```python
from build123d import *

# Parameters (mm, degrees)
SKETCH5_W           = 101.6
SKETCH5_H           = 101.6
SKETCH5_W_2         = 20.32
SKETCH5_H_2         = 20.32
BOSS_EXTRUDE1_DEPTH = 228.6
SKETCH6_R           = 41.91
CUT_EXTRUDE1_DEPTH  = 127
SKETCH5_3_W         = 20.32
SKETCH5_3_H         = 20.32
CUT_EXTRUDE2_DEPTH  = 25.4
CUT_EXTRUDE3_DEPTH  = 76.2
SKETCH9_R           = 7.62
CUT_EXTRUDE4_DEPTH  = 56.642


with BuildPart() as part:
    # Sketch5 → Boss-Extrude1 (new body)
    # profile 1 of 5: a face of its own
    with BuildSketch(Plane(origin=(0, 0, 0), x_dir=(1, 0, 0), z_dir=(0, 1, 0))):
        with Locations((50.8, 50.8)):
            Rectangle(SKETCH5_W, SKETCH5_H)
        with Locations((16.51, 15.457317153)):
            Rectangle(SKETCH5_W_2, SKETCH5_H_2, mode=Mode.SUBTRACT)
        with Locations((85.09, 15.457317153)):
            Rectangle(SKETCH5_W_2, SKETCH5_H_2, mode=Mode.SUBTRACT)
        with Locations((85.09, 85.09)):
            Rectangle(SKETCH5_W_2, SKETCH5_H_2, mode=Mode.SUBTRACT)
        with Locations((16.51, 85.09)):
            Rectangle(SKETCH5_W_2, SKETCH5_H_2, mode=Mode.SUBTRACT)
    # profile 2 of 5: a face of its own
    with BuildSketch(Plane(origin=(0, 0, 0), x_dir=(1, 0, 0), z_dir=(0, 1, 0))):
        with Locations((85.09, 15.457317153)):
            Rectangle(SKETCH5_W_2, SKETCH5_H_2)
    # profile 3 of 5: a face of its own
    with BuildSketch(Plane(origin=(0, 0, 0), x_dir=(1, 0, 0), z_dir=(0, 1, 0))):
        with Locations((85.09, 85.09)):
            Rectangle(SKETCH5_W_2, SKETCH5_H_2)
    # profile 4 of 5: a face of its own
    with BuildSketch(Plane(origin=(0, 0, 0), x_dir=(1, 0, 0), z_dir=(0, 1, 0))):
        with Locations((16.51, 15.457317153)):
            Rectangle(SKETCH5_W_2, SKETCH5_H_2)
    # profile 5 of 5: a face of its own
    with BuildSketch(Plane(origin=(0, 0, 0), x_dir=(1, 0, 0), z_dir=(0, 1, 0))):
        with Locations((16.51, 85.09)):
            Rectangle(SKETCH5_W_2, SKETCH5_H_2)
    extrude(amount=BOSS_EXTRUDE1_DEPTH)

    # Sketch6 → Cut-Extrude1 (cut)
    with BuildSketch(Plane(origin=(0, 0, 0), x_dir=(1, 0, 0), z_dir=(0, 1, 0))):
        with Locations(Location((50.8, 50.8, 0), (0, 0, 270))):
            Circle(SKETCH6_R)
    extrude(amount=CUT_EXTRUDE1_DEPTH, mode=Mode.SUBTRACT)

    # Sketch5_3 → Cut-Extrude2 (cut)
    with BuildSketch(Plane(origin=(0, 0, 0), x_dir=(1, 0, 0), z_dir=(0, 1, 0))):
        with Locations((16.51, 15.457317153)):
            Rectangle(SKETCH5_3_W, SKETCH5_3_H)
        with Locations((85.09, 15.457317153)):
            Rectangle(SKETCH5_3_W, SKETCH5_3_H)
        with Locations((85.09, 85.09)):
            Rectangle(SKETCH5_3_W, SKETCH5_3_H)
        with Locations((16.51, 85.09)):
            Rectangle(SKETCH5_3_W, SKETCH5_3_H)
    extrude(amount=CUT_EXTRUDE2_DEPTH, mode=Mode.SUBTRACT)

    # Sketch7 → Cut-Extrude3 (cut)
    with BuildSketch(Plane(origin=(0, 220.98, 0), x_dir=(1, 0, 0), z_dir=(0, 1, 0))):
        with BuildLine():
            Line((76.2, 50.8), (76.2, -137.296764807))
            Line((76.2, -137.296764807), (25.4, -137.296764807))
            Line((25.4, -137.296764807), (25.4, 50.8))
            ThreePointArc((25.4, 50.8), (50.8, 76.2), (76.2, 50.8))
        make_face()
    extrude(amount=-CUT_EXTRUDE3_DEPTH, mode=Mode.SUBTRACT)

    # Sketch9 → Cut-Extrude4 (cut)
    with BuildSketch(Plane.XY):
        with Locations((50.8, 114.3)):
            Circle(SKETCH9_R)
        with Locations((50.8, 88.9)):
            Circle(SKETCH9_R)
    extrude(amount=-CUT_EXTRUDE4_DEPTH, mode=Mode.SUBTRACT)


solid = part.part
```
Check sheet for the modelled part. Datum: model origin and axes. Units: mm. A direction names the side the tool comes from. Give positions to 0.01 mm unless a question says otherwise; leave off trailing zeros. Loops run counter-clockwise (first coordinate to the right, second up) from the corner with the lowest first, then second, coordinate; pieces in that order, holes last. Notation, with made-up numbers: (76, 54) - (97, 54) arc R18 ccw to (97, 66) - close; hole circle Ø8 at (55, 32). An arc over 180 degrees is marked (long way). One line per question, with ' | ' between items. Start each with the question number.
1. Gauge pin test, flat ends, axial feed: pin 1 Ø22.5 at (x, z) = (15.5, -88) entering from -Y; pin 2 Ø1.5 at (x, y) = (60.5, 181.5) entering from +Z. Record the tip position at first contact, or that the pin passes through.
2. Set-up check for faces 1 (the flat face through (6.35, 13, -15)), 2 (the flat face through (51, 220.98, -39)): record each of +Z, -Z, +X, -X, +Y, -Y from which the full face is reachable in a straight line by a thin tool's end or side.
3. Cross-section at C-C, the plane y = 114.3. Enter the section's corners in (x, z).
4. Cross-section at B-B, the plane y = 75.5. Enter the section's corners in (x, z).
5. Draft check along Y on faces 3 (the flat face through (51, 127, -51)), 4 (the cylindrical face through (58.068, 116.589, -4.727)), 5 (the flat face through (61, 87, 0)), 6 (the flat face through (50, 228.6, -52)). Enter one of: released by +Y, released by -Y, zero draft, split by the parting line, or undercut.
6. Material ranges on line 1 along X through (y, z) = (22, -94.5); line 2 along X through (y, z) = (174, -23); line 3 along Y through (x, z) = (64, -67), recorded low to high. Write a range as [from, to].
7. Cross-section at D-D, the plane x = 23. Enter the section's corners in (y, z), plus the area to 3 significant figures.
8. Cross-section at A-A, the plane x = 50.8. Enter the section's corners in (y, z).
Check result:
1) pin 1: stops at y = 0 | pin 2: stops at z = -73.95
2) face 1: -Y | face 2: +Z
3) outline: (0, -101.6) - (101.6, -101.6) - (101.6, 0) - (58.42, 0) - (58.42, -9.59) arc R41.91 cw (long way) to (43.18, -9.59) - (43.18, 0) - (0, 0) - close
4) outline: (0, -101.6) - (101.6, -101.6) - (101.6, 0) - (0, 0) - close; hole circle Ø83.82 at (50.8, -50.8)
5) face 3: released by -Y | face 4: undercut | face 5: zero draft | face 6: released by +Y
6) line 1: x = [0, 6.35], [26.67, 74.93], [95.25, 101.6] | line 2: x = [0, 25.4], [76.2, 101.6] | line 3: y = [127, 144.78], [220.98, 228.6]
7) outline: (0, -101.6) - (228.6, -101.6) - (228.6, 0) - (0, 0) - (0, -5.3) - (25.4, -5.3) - (25.4, -19.44) - (127, -19.44) - (127, -82.16) - (25.4, -82.16) - (25.4, -95.25) - (0, -95.25) - close | area: 14,600 mm2
8) outline: (0, -101.6) - (228.6, -101.6) - (228.6, 0) - (220.98, 0) - (220.98, -76.2) - (144.78, -76.2) - (144.78, 0) - (121.92, 0) - (121.92, -8.89) - (127, -8.89) - (127, -92.71) - (0, -92.71) - close; (0, -8.89) - (81.28, -8.89) - (81.28, 0) - (0, 0) - close; (96.52, -8.89) - (106.68, -8.89) - (106.68, 0) - (96.52, 0) - close
